```python
from build123d import *

# Parameters (mm, degrees)
SKETCH029_W             = 70
SKETCH029_H             = 7.62
SKETCH029_R             = 1
PAD017_DEPTH            = 1.1
SKETCH033_R             = 2.5
PAD021_DEPTH            = 8
PAD015_DEPTH            = 1.5
BODY007_PLACEMENT_ANGLE = 180


with BuildPart() as part:
    # Sketch029 → Pad017 (new body)
    with BuildSketch(Plane.XY):
        with Locations((35, 3.81)):
            Rectangle(SKETCH029_W, SKETCH029_H)
        with Locations((34, 5.08)):
            Circle(SKETCH029_R, mode=Mode.SUBTRACT)
    extrude(amount=PAD017_DEPTH)

    # Sketch033 (on Face7 of Pad017) → Pad021 (join)
    with BuildSketch(Plane.XY.offset(1.1)):
        with Locations((26.38, 3.81)):
            Circle(SKETCH033_R)
        with Locations((41.62, 3.81)):
            Circle(SKETCH033_R)
        with Locations((59.4, 3.81)):
            Circle(SKETCH033_R)
        with Locations((8.6, 3.81)):
            Circle(SKETCH033_R)
    extrude(amount=PAD021_DEPTH)

    # Sketch025 (on Face5 of Pad021) → Pad015 (join)
    with BuildSketch(Plane.XY.offset(1.1)):
        Polygon((3.106141, 4.536354), (3.106141, 5.623646), (2.164519, 6.167292), (1.222896, 5.623646), (1.222896, 4.536354), (2.164519, 3.992708), align=None)
    extrude(amount=PAD015_DEPTH)


with BuildPart() as part_1:
    # Body007 placement: moved
    add(part.part.moved(Location((75, 71, 0))).rotate(Axis((75, 71, 0), (0, 0, 1)), BODY007_PLACEMENT_ANGLE))


solid = part_1.part
```
Input: part model. Units: mm. Frame: model coordinates. A direction names the side the tool comes from. Give positions to 0.01 mm unless a question says otherwise; leave off trailing zeros. Order: outer loops, then holes, each group sorted by start corner. A loop starts at its lowest first (then second) coordinate and runs counter-clockwise, first axis right, second up.
1. Cut plane B-B (x = 15.6). Return loops of the section in (y, z).
Computed:
outline: (63.38, 0) - (71, 0) - (71, 1.1) - (69.69, 1.1) - (69.69, 9.1) - (64.69, 9.1) - (64.69, 1.1) - (63.38, 1.1) - close
2. Draft query along Y for faces 1 (the face through (64.09, 68.15, 5.04)), 2 (the face through (5, 67.2, 0.5)), 3 (the face through (40.046, 65.62, 0.542)), 4 (the face through (40.5, 71, 0.5)). Return one class per face: released by +Y, released by -Y, zero draft, split by the parting line, or undercut.
Computed:
face 1: split by the parting line
face 2: zero draft
face 3: undercut
face 4: released by +Y
3. Set-up query: faces 5 (the face through (73.777, 66, 2)), 6 (the face through (71.894, 66, 2)), 7 (the face through (35.364, 68.711, 5.044)), 8 (the face through (66, 67, 9.1)), 9 (the face through (75, 67.2, 0.5)). Return all of +Z, -Z, +X, -X, +Y, -Y with unobstructed straight access to the full face (end or side cutting, diameter ignored); none if empty.
Computed:
face 5: +Z, +X, +Y, -Y
face 6: +Z, +Y, -Y
face 7: +Z
face 8: +Z, +X, -X, +Y, -Y
face 9: +Z, -Z, +X, +Y, -Y
4. Pin query (flat end, axial travel): pin 1 Ø1 at (x, z) = (26.5, 1.5) entering from -Y; pin 2 Ø1.5 at (x, z) = (46, 2.5) entering from +Y; pin 3 Ø3 at (y, z) = (65.5, 3) entering from -X; pin 4 Ø1.5 at (x, y) = (72.5, 66) entering from +Z. Return the tip coordinate at first contact, or that it passes through.
Computed:
pin 1: stops at y = 63.38
pin 2: stops at y = 68.85
pin 3: stops at x = 13.11
pin 4: stops at z = 2.6
5. Cut plane A-A (x = 41). Return loops of the section in (y, z), and give its area (3 significant figures).
Computed:
outline: (63.38, 0) - (64.92, 0) - (64.92, 1.1) - (63.38, 1.1) - close; (66.92, 0) - (71, 0) - (71, 1.1) - (66.92, 1.1) - close
area: 6.18 mm2
6. Cut plane C-C (z = 5.25). Return loops of the section in (x, y).
Computed:
outline: circle Ø5 at (15.6, 67.19); circle Ø5 at (33.38, 67.19); circle Ø5 at (48.62, 67.19); circle Ø5 at (66.4, 67.19)
7. Cut plane D-D (x = 64.5). Return loops of the section in (y, z), and give its area (3 significant figures).
Computed:
outline: (63.38, 0) - (71, 0) - (71, 1.1) - (68.81, 1.1) - (68.81, 9.1) - (65.57, 9.1) - (65.57, 1.1) - (63.38, 1.1) - close
area: 34.4 mm2
8. Line query: probe 1 along X at (y, z) = (65.92, 0.9); probe 2 along Y at (x, z) = (41, 0.5); probe 3 along X at (y, z) = (67.5, 3.75). Output: solid intervals per line, ascending.
Computed:
probe 1: x = 5 to 40, 42 to 75
probe 2: y = 63.38 to 64.92, 66.92 to 71
probe 3: x = 13.12 to 18.08, 30.9 to 35.86, 46.14 to 51.1, 63.92 to 68.88
